For this review, take the finished solid that the model builds, in its own axes (mm). A direction names the side the tool comes from. Round coordinates to 2 decimals unless told otherwise and drop trailing zeros. Order: outer loops, then holes, each group sorted by start corner. A loop starts at its lowest first (then second) coordinate and runs counter-clockwise, first axis right, second up. Notation, with made-up numbers: (64.5, -33) -> (70.5, -33) arc R27 ccw to (70.5, 5) -> close; hole circle Ø9 at (-25, -36). An arc over 180 degrees is marked (long way). Answer in a Markdown table with one row per item.
```python
from build123d import *

# Parameters (mm, degrees)
PAD_DEPTH         = 20
FILLET_R          = 11
FILLET001_R       = 5
THICKNESS_T       = -1.8
SKETCH001_W       = 1.5
SKETCH001_H       = 20
PAD001_DEPTH      = 7
POCKET_DEPTH      = 1.801
POCKET_DEPTH_BACK = 18.201


with BuildPart() as part:
    # Sketch → Pad (new body)
    with BuildSketch(Plane.XY):
        Polygon((0, 0), (18, 0), (18, -10), (-7.339746, -18), (-16, -13), (0, -5), align=None)
    extrude(amount=PAD_DEPTH)

    # Fillet
    fillet_edges = [part.edges().sort_by_distance(p)[0] for p in [
        (18, -10, 10),
    ]]
    fillet(fillet_edges, radius=FILLET_R)

    # Fillet001
    fillet001_edges = [part.edges().sort_by_distance(p)[0] for p in [
        (0, -5, 10),
    ]]
    fillet(fillet001_edges, radius=FILLET001_R)

    # Thickness
    thickness_openings = [part.faces().sort_by_distance(p)[0] for p in [
        (9, 0, 10),
        (-11.669873, -15.5, 10),
    ]]
    offset(amount=THICKNESS_T, openings=thickness_openings)

    # Sketch001 → Pad001 (new body)
    with BuildSketch(Plane(origin=(0, 0, 0), x_dir=(-1, 0, 0), z_dir=(0, 1, 0))):
        with Locations((-17.25, 10)):
            Rectangle(SKETCH001_W, SKETCH001_H)
        with Locations((-0.75, 10)):
            Rectangle(SKETCH001_W, SKETCH001_H)
    extrude(amount=PAD001_DEPTH)

    # Sketch002 → Pocket (cut, two sides)
    with BuildSketch(Plane.XY.offset(1.8)) as pocket_sk:
        Polygon((-14.132027, -14.078475), (-9.826848, -11.925885), (-4.388537, -15.1807), (-9.45335, -16.77971), align=None)
    extrude(amount=-POCKET_DEPTH, mode=Mode.SUBTRACT)
    extrude(pocket_sk.sketch, amount=POCKET_DEPTH_BACK, mode=Mode.SUBTRACT)


solid = part.part
```
Q1. Take a section at C-C, the plane x = -1. Write out the cut boundary in (y, z), then the cut area to 3 significant figures.
Answer key:
| item | result |
|---|---|
| outline | (-16, 0) -> (-4.91, 0) -> (-4.91, 20) -> (-16, 20) -> close; hole (-14.11, 1.8) -> (-7.41, 1.8) -> (-7.41, 18.2) -> (-14.11, 18.2) -> close |
| area | 112 mm^2 |
Q2. To check wall thickness, follow probe 1 along X at (y, z) = (1.25, 1.5); probe 2 along Z at (x, y) = (14.5, -4.75); probe 3 along X at (y, z) = (-0.25, 14). State the ranges of each line that lie inside material, in increasing order.
Answer key:
| item | result |
|---|---|
| probe 1 | x = 0 to 1.5, 16.5 to 18 |
| probe 2 | z = 0 to 1.8, 18.2 to 20 |
| probe 3 | x = 0 to 1.8, 16.2 to 18 |
Q3. Take a section at B-B, the plane y = 2.75. Write out the cut boundary in (x, z), then the cut area to 3 significant figures.
Answer key:
| item | result |
|---|---|
| outline | (0, 0) -> (1.5, 0) -> (1.5, 20) -> (0, 20) -> close; (16.5, 0) -> (18, 0) -> (18, 20) -> (16.5, 20) -> close |
| area | 60.0 mm^2 |
Q4. Tool access review of faces 1 (the face through (6, -7, 18.2)), 2 (the face through (14.47, -7.31, 10.11)), 3 (the face through (-7.15, -13.53, 0.91)), 4 (the face through (1.5, 3, 10)): name each direction out of +Z, -Z, +X, -X, +Y, -Y from which nothing blocks a thin tool from reaching the whole face with its end or side.
Answer key:
| item | result |
|---|---|
| face 1 | none |
| face 2 | +Y |
| face 3 | +Z, -Z |
| face 4 | +Z, -Z, +Y |
Q5. The part is to be moulded in two halves that separate along Z. For faces 5 (the face through (6, -7, 1.8)), 6 (the face through (0, 2, 10)), 7 (the face through (5, -6, 0)), 8 (the face through (0.81, -5.44, 10.11)), say which applies: +Z half, -Z half, draft (parallel to the pull), parting line (faces both ways), or undercut.
Answer key:
| item | result |
|---|---|
| face 5 | undercut |
| face 6 | draft |
| face 7 | -Z half |
| face 8 | undercut |
Q6. Clearance check with flat-ended pins moving along their axes: pin 1 Ø4.5 at (x, y) = (6, -6.5) entering from -Z; pin 2 Ø0.6 at (y, z) = (-0.5, 10) entering from -X; pin 3 Ø3 at (x, z) = (-10.5, 15) entering from -Y; pin 4 Ø1.5 at (y, z) = (-6.5, 12.5) entering from +X. State where each tip first meets the part, or that it passes through.
Answer key:
| item | result |
|---|---|
| pin 1 | stops at z = 0 |
| pin 2 | stops at x = 0 |
| pin 3 | stops at y = -17.04 |
| pin 4 | stops at x = 17.32 |
